```python
from build123d import *

# Parameters (mm, degrees)
SKETCH_1_R               = 4
EXTRUDE_1_DEPTH          = 9
SKETCH_2_R               = 26
EXTRUDE_2_DEPTH          = 35
SKETCH_3_R               = 40
EXTRUDE_3_DEPTH          = 9
HOLE_WIZARD_M8_1_D       = 6.8
HOLE_WIZARD_M8_1_DEPTH   = 9
PATTERN_CIRCULAR_1_COUNT = 6
SKETCH_6_R               = 20
CUT_EXTRUDE_1_DEPTH      = 100.700603114
SKETCH_7_R               = 37.5
CUT_EXTRUDE_2_DEPTH      = 6
SKETCH_8_R               = 1.5
CUT_EXTRUDE_3_DEPTH      = 100.700603114


with BuildPart() as part:
    # 草图1 → 凸台-拉伸1 (new body)
    with BuildSketch(Plane(origin=(0, 0, 0), x_dir=(1, 0, 0), z_dir=(0, 1, 0))):
        with BuildLine():
            Line((-18.734993995, 57), (18.734993995, 57))
            ThreePointArc((18.734993995, 57), (59.760164517, -5.359359749), (8.293957962, -59.423987255))
            ThreePointArc((8.293957962, -59.423987255), (0, -54.527427418), (-8.293957962, -59.423987255))
            ThreePointArc((-8.293957962, -59.423987255), (-59.760164517, -5.359359749), (-18.734993995, 57))
        make_face()
        with Locations(Location((-48.041735691, 19.899538483, 0), (0, 0, 270))):
            Circle(SKETCH_1_R, mode=Mode.SUBTRACT)
        with Locations(Location((-19.899538483, 48.041735691, 0), (0, 0, 270))):
            Circle(SKETCH_1_R, mode=Mode.SUBTRACT)
        with Locations(Location((19.899538483, 48.041735691, 0), (0, 0, 270))):
            Circle(SKETCH_1_R, mode=Mode.SUBTRACT)
        with Locations(Location((48.041735691, 19.899538483, 0), (0, 0, 270))):
            Circle(SKETCH_1_R, mode=Mode.SUBTRACT)
        with Locations(Location((48.041735691, -19.899538483, 0), (0, 0, 270))):
            Circle(SKETCH_1_R, mode=Mode.SUBTRACT)
        with Locations(Location((19.899538483, -48.041735691, 0), (0, 0, 270))):
            Circle(SKETCH_1_R, mode=Mode.SUBTRACT)
        with Locations(Location((-19.899538483, -48.041735691, 0), (0, 0, 270))):
            Circle(SKETCH_1_R, mode=Mode.SUBTRACT)
        with Locations(Location((-48.041735691, -19.899538483, 0), (0, 0, 270))):
            Circle(SKETCH_1_R, mode=Mode.SUBTRACT)
    extrude(amount=EXTRUDE_1_DEPTH)

    # 草图2 → 凸台-拉伸2 (add)
    with BuildSketch(Plane(origin=(0, 9, 0), x_dir=(1, 0, 0), z_dir=(0, 1, 0))):
        with Locations(Location((0, 0, 0), (0, 0, 270))):
            Circle(SKETCH_2_R)
    extrude(amount=EXTRUDE_2_DEPTH)

    # 草图3 → 凸台-拉伸3 (add)
    with BuildSketch(Plane(origin=(0, 44, 0), x_dir=(1, 0, 0), z_dir=(0, 1, 0))):
        with Locations(Location((0, 0, 0), (0, 0, 270))):
            Circle(SKETCH_3_R)
    extrude(amount=EXTRUDE_3_DEPTH)

    # M8 螺纹孔1
    with Locations(Plane(origin=(0, 53, 0), x_dir=(1, 0, 0), z_dir=(0, 1, 0))):
        with Locations((0, 31.5)):
            hole_wizard_m8_1 = Hole(HOLE_WIZARD_M8_1_D / 2, depth=HOLE_WIZARD_M8_1_DEPTH)

    # 阵列(圆周)1: M8 螺纹孔1 ×6 about axis
    pattern_circular_1_axis = Axis((0, 0, 0), (0, 1, 0))
    for i in range(1, PATTERN_CIRCULAR_1_COUNT):
        add(hole_wizard_m8_1.rotate(pattern_circular_1_axis, i * 360 / PATTERN_CIRCULAR_1_COUNT), mode=Mode.SUBTRACT)

    # 草图6 → 切除-拉伸1 (cut, through all)
    with BuildSketch(Plane(origin=(0, 53, 0), x_dir=(1, 0, 0), z_dir=(0, 1, 0))):
        with Locations(Location((0, 0, 0), (0, 0, 270))):
            Circle(SKETCH_6_R)
    extrude(amount=-CUT_EXTRUDE_1_DEPTH, mode=Mode.SUBTRACT)

    # 草图7 → 切除-拉伸2 (cut)
    with BuildSketch(Plane.XZ):
        with Locations(Location((0, 0, 0), (0, 0, 270))):
            Circle(SKETCH_7_R)
    extrude(amount=-CUT_EXTRUDE_2_DEPTH, mode=Mode.SUBTRACT)

    # 草图8 → 切除-拉伸3 (cut, through all)
    with BuildSketch(Plane(origin=(0, 53, 0), x_dir=(1, 0, 0), z_dir=(0, 1, 0))):
        with Locations(Location((0, 31.5, 0), (0, 0, 270))):
            Circle(SKETCH_8_R)
    extrude(amount=-CUT_EXTRUDE_3_DEPTH, mode=Mode.SUBTRACT)


solid = part.part
```
For this review, take the finished solid that the model builds, in its own axes (mm). A direction names the side the tool comes from. Coordinates: 2 decimals unless noted, no trailing zeros. Write each loop counter-clockwise with the first axis right and the second up, starting at its lowest first coordinate (ties: lowest second). Pieces come first, ordered by that corner, then holes.
(1) For pin 1 Ø6 at (x, z) = (27.28, -15.75) entering from +Y; pin 2 Ø8 at (x, z) = (27.28, 15.75) entering from +Y; pin 3 Ø9 at (x, z) = (0, 31.5) entering from -Y; pin 4 Ø2 at (y, z) = (8, 35.5) entering from -X, all flat-tipped, find the tip position at first contact; note any pin that passes through.
(2) Tool access review of faces 1 (the face through (0.74, 48.44, -28.18)), 2 (the face through (-22.818, 2.958, 29.759)), 3 (the face through (0.8, 9, 26.3)), 4 (the face through (21.101, 4.437, -44.226)): name each direction out of +Z, -Z, +X, -X, +Y, -Y from which nothing blocks a thin tool from reaching the whole face with its end or side.
(3) Add section A-A on x = 0. Count the separate pieces of the cut face and the enclosed holes in it, then the cut area to 3 significant figures.
(4) Add section B-B on z = 0. Give the boundary of the cut face in (x, y), then the cut area to 3 significant figures.
(5) Add section C-C on z = 22. Give the boundary of the cut face in (x, y).
(6) Add section D-D on y = 47.5. Give the boundary of the cut face in (x, z), then the cut area to 3 significant figures.
(7) Wall thickness on probe 1 along X at (y, z) = (4.7, 0); probe 2 along Y at (x, z) = (25, -3.5); probe 3 along Y at (x, z) = (-6.5, -28): over which ranges is each line inside the solid? List them lowest first.
(8) The part is to be moulded in two halves that separate along Y. For faces 5 (the face through (-0.74, 48.44, 28.18)), 6 (the face through (-15.821, 26.255, -20.633)), 7 (the face through (-16, 6, -16)), say which applies: +Y half, -Y half, draft (parallel to the pull), parting line (faces both ways), or undercut.
Answer sheet:
1. pin 1: stops at y = 9
1. pin 2: stops at y = 53
1. pin 3: stops at y = 6
1. pin 4: stops at x = -49.09
2. face 1: +Y
2. face 2: -Y
2. face 3: none
2. face 4: +Y, -Y
3. separate pieces: 5
3. enclosed holes: 0
3. area: 1,080 mm2
4. outline: (-60, 0) - (-37.5, 0) - (-37.5, 6) - (-20, 6) - (-20, 53) - (-40, 53) - (-40, 44) - (-26, 44) - (-26, 9) - (-60, 9) - close; (20, 6) - (37.5, 6) - (37.5, 0) - (60, 0) - (60, 9) - (26, 9) - (26, 44) - (40, 44) - (40, 53) - (20, 53) - close
4. area: 1,290 mm2
5. outline: (-55.82, 0) - (-51.45, 0) - (-51.45, 9) - (-55.82, 9) - close; (-44.64, 0) - (-30.37, 0) - (-30.37, 6) - (30.37, 6) - (30.37, 0) - (44.64, 0) - (44.64, 9) - (13.86, 9) - (13.86, 44) - (33.41, 44) - (33.41, 53) - (-33.41, 53) - (-33.41, 44) - (-13.86, 44) - (-13.86, 9) - (-44.64, 9) - close; (51.45, 0) - (55.82, 0) - (55.82, 9) - (51.45, 9) - close
6. outline: circle Ø80 at (0, 0); hole circle Ø6.8 at (-27.28, -15.75); hole circle Ø6.8 at (-27.28, 15.75); hole circle Ø40 at (0, 0); hole circle Ø6.8 at (0, -31.5); hole circle Ø6.8 at (0, 31.5); hole circle Ø6.8 at (27.28, -15.75); hole circle Ø6.8 at (27.28, 15.75)
6. area: 3,550 mm2
7. probe 1: x = -60 to -37.5, 37.5 to 60
7. probe 2: y = 6 to 53
7. probe 3: y = 6 to 9, 44 to 53
8. face 5: draft
8. face 6: undercut
8. face 7: -Y half
